```python
from build123d import *

# Parameters (mm, degrees)
SKETCH1_W           = 60
SKETCH1_H           = 54
BOSS_EXTRUDE1_DEPTH = 38
SKETCH2_W           = 44
SKETCH2_H           = 52
CUT_EXTRUDE1_DEPTH  = 19
SKETCH3_W           = 35
SKETCH3_H           = 52
CUT_EXTRUDE2_DEPTH  = 18
SKETCH4_W           = 6
SKETCH4_H           = 10
CUT_EXTRUDE3_DEPTH  = 38
SKETCH5_W           = 14
SKETCH5_H           = 52
CUT_EXTRUDE5_DEPTH  = 15
SKETCH6_W           = 13
SKETCH6_H           = 52
CUT_EXTRUDE6_DEPTH  = 4
SKETCH8_W           = 15
SKETCH8_H           = 13
CUT_EXTRUDE7_DEPTH  = 6
SKETCH10_W          = 13
SKETCH10_H          = 5
CUT_EXTRUDE8_DEPTH  = 6
SKETCH11_W          = 4
SKETCH11_H          = 5
CUT_EXTRUDE9_DEPTH  = 3
SKETCH12_W          = 5
SKETCH12_H          = 2
CUT_EXTRUDE10_DEPTH = 13
CUT_EXTRUDE11_DEPTH = 1
SKETCH14_W          = 13
SKETCH14_H          = 1
BOSS_EXTRUDE2_DEPTH = 4
SKETCH15_W          = 13
SKETCH15_H          = 1
BOSS_EXTRUDE3_DEPTH = 4


with BuildPart() as part:
    # Sketch1 → Boss-Extrude1 (new body)
    with BuildSketch(Plane(origin=(0, 0, 0), x_dir=(1, 0, 0), z_dir=(0, 1, 0))):
        with Locations((-83.874465942, -33.946435202)):
            Rectangle(SKETCH1_W, SKETCH1_H)
    extrude(amount=BOSS_EXTRUDE1_DEPTH)

    # Sketch2 → Cut-Extrude1 (cut)
    with BuildSketch(Plane(origin=(0, 38, 0), x_dir=(1, 0, 0), z_dir=(0, 1, 0))):
        with Locations((-76.874465942, -33.946435202)):
            Rectangle(SKETCH2_W, SKETCH2_H)
    extrude(amount=-CUT_EXTRUDE1_DEPTH, mode=Mode.SUBTRACT)

    # Sketch3 → Cut-Extrude2 (cut)
    with BuildSketch(Plane(origin=(0, 0, 0), x_dir=(-1, 0, 0), z_dir=(0, -1, 0))):
        with Locations((95.374465942, -33.946435202)):
            Rectangle(SKETCH3_W, SKETCH3_H)
    extrude(amount=-CUT_EXTRUDE2_DEPTH, mode=Mode.SUBTRACT)

    # Sketch4 → Cut-Extrude3 (cut)
    with BuildSketch(Plane(origin=(0, 18, 0), x_dir=(-1, 0, 0), z_dir=(0, -1, 0))):
        with Locations((108.874465942, -34.946435202)):
            Rectangle(SKETCH4_W, SKETCH4_H)
    extrude(amount=-CUT_EXTRUDE3_DEPTH, mode=Mode.SUBTRACT)

    # Sketch5 → Cut-Extrude5 (cut)
    with BuildSketch(Plane(origin=(0, 38, 0), x_dir=(1, 0, 0), z_dir=(0, 1, 0))):
        with Locations((-105.874465942, -33.946435202)):
            Rectangle(SKETCH5_W, SKETCH5_H)
    extrude(amount=-CUT_EXTRUDE5_DEPTH, mode=Mode.SUBTRACT)

    # Sketch6 → Cut-Extrude6 (cut)
    with BuildSketch(Plane(origin=(0, 23, 0), x_dir=(1, 0, 0), z_dir=(0, 1, 0))):
        with Locations((-106.374465942, -33.946435202)):
            Rectangle(SKETCH6_W, SKETCH6_H)
    extrude(amount=-CUT_EXTRUDE6_DEPTH, mode=Mode.SUBTRACT)

    # Sketch8 → Cut-Extrude7 (cut)
    with BuildSketch(Plane(origin=(0, 0, 0), x_dir=(-1, 0, 0), z_dir=(0, -1, 0))):
        with Locations((65.874465942, -17.946435202)):
            Rectangle(SKETCH8_W, SKETCH8_H)
    extrude(amount=-CUT_EXTRUDE7_DEPTH, mode=Mode.SUBTRACT)

    # Sketch10 → Cut-Extrude8 (cut)
    with BuildSketch(Plane(origin=(-73.374465942, 0, 0), x_dir=(0, 0, -1), z_dir=(1, 0, 0))):
        with Locations((-17.946435202, 3.5)):
            Rectangle(SKETCH10_W, SKETCH10_H)
    extrude(amount=-CUT_EXTRUDE8_DEPTH, mode=Mode.SUBTRACT)

    # Sketch11 → Cut-Extrude9 (cut)
    with BuildSketch(Plane.XZ):
        with Locations((-65.874465942, 48.446435202)):
            Rectangle(SKETCH11_W, SKETCH11_H)
    extrude(amount=-CUT_EXTRUDE9_DEPTH, mode=Mode.SUBTRACT)

    # Sketch12 → Cut-Extrude10 (cut)
    with BuildSketch(Plane(origin=(-67.874465942, 0, 0), x_dir=(0, 0, -1), z_dir=(1, 0, 0))):
        with Locations((-48.446435202, 2)):
            Rectangle(SKETCH12_W, SKETCH12_H)
    extrude(amount=-CUT_EXTRUDE10_DEPTH, mode=Mode.SUBTRACT)

    # Sketch13 → Cut-Extrude11 (cut)
    with BuildSketch(Plane.ZY.offset(113.874465942)):
        with BuildLine():
            Line((32.733045904, 15), (32.733045904, 22))
            ThreePointArc((32.733045904, 22), (35.233045904, 24.5), (37.733045904, 22))
            Line((37.733045904, 22), (37.733045904, 15))
            ThreePointArc((37.733045904, 15), (35.233045904, 12.5), (32.733045904, 15))
        make_face()
    extrude(amount=-CUT_EXTRUDE11_DEPTH, mode=Mode.SUBTRACT)

    # Sketch14 → Boss-Extrude2 (add)
    with BuildSketch(Plane(origin=(0, 19, 0), x_dir=(1, 0, 0), z_dir=(0, 1, 0))):
        with Locations((-106.374465942, -40.446435202)):
            Rectangle(SKETCH14_W, SKETCH14_H)
    extrude(amount=BOSS_EXTRUDE2_DEPTH)

    # Sketch15 → Boss-Extrude3 (add)
    with BuildSketch(Plane(origin=(0, 19, 0), x_dir=(1, 0, 0), z_dir=(0, 1, 0))):
        with Locations((-106.374465942, -29.446435202)):
            Rectangle(SKETCH15_W, SKETCH15_H)
    extrude(amount=BOSS_EXTRUDE3_DEPTH)


solid = part.part
```
Work out the finished part from the listing and answer in its coordinate system (mm). A direction names the side the tool comes from. Give positions to 0.01 mm unless a question says otherwise; leave off trailing zeros. Order: outer loops, then holes, each group sorted by start corner. A loop starts at its lowest first (then second) coordinate and runs counter-clockwise, first axis right, second up. Notation, with made-up numbers: M 61.25,50 L 95.25,50 A20 ccw 95.25,56 Z; hole C -39,-15.75 d7. An arc over 180 degrees is marked long. Return JSON: item names as keys, results as strings.
1) Section C-C, the plane y = 27 is taken. Write down the section's boundary in (x, z).
Resolved:
{"outline": "M -113.87,6.95 L -53.87,6.95 L -53.87,60.95 L -113.87,60.95 Z; hole M -112.87,7.95 L -54.87,7.95 L -54.87,59.95 L -112.87,59.95 Z"}
2) Section D-D, the plane x = -79 is taken. Write down the section's boundary in (y, z).
Resolved:
{"outline": "M 0,6.95 L 38,6.95 L 38,7.95 L 19,7.95 L 19,59.95 L 38,59.95 L 38,60.95 L 0,60.95 L 0,59.95 L 18,59.95 L 18,7.95 L 0,7.95 Z"}
3) Section A-A, the plane z = 32 is taken. Write down the section's boundary in (x, y).
Resolved:
{"outline": "M -113.87,0 L -112.87,0 L -112.87,18 L -111.87,18 L -111.87,19 L -112.87,19 L -112.87,38 L -113.87,38 Z; M -105.87,18 L -77.87,18 L -77.87,0 L -53.87,0 L -53.87,38 L -54.87,38 L -54.87,19 L -98.87,19 L -98.87,23 L -99.87,23 L -99.87,19 L -105.87,19 Z"}
4) A tool of negligible diameter and unlimited length cuts with its end or side. For faces 5 (the flat face through (-99.874, 21, 19)), 6 (the flat face through (-71, 2, 50.946)), 7 (the flat face through (-77.874, 9, 34)), from which of +Z, -Z, +X, -X, +Y, -Y can it reach the whole face along a straight path? Write none if from no direction.
Resolved:
{"face 5": "+Y", "face 6": "none", "face 7": "-Y"}
5) Section B-B, the plane y = 21 is taken. Write down the section's boundary in (x, z), plus the area to 3 significant figures.
Resolved:
{"outline": "M -113.87,6.95 L -53.87,6.95 L -53.87,60.95 L -113.87,60.95 L -113.87,37.73 L -112.87,37.73 L -112.87,39.95 L -99.87,39.95 L -99.87,29.95 L -112.87,29.95 L -112.87,32.73 L -113.87,32.73 Z; hole M -112.87,7.95 L -99.87,7.95 L -99.87,28.95 L -112.87,28.95 Z; hole M -112.87,40.95 L -99.87,40.95 L -99.87,59.95 L -112.87,59.95 Z; hole M -98.87,7.95 L -54.87,7.95 L -54.87,59.95 L -98.87,59.95 Z", "area": "297 mm^2"}
6) Straight lines are drawn through the part: line 1 along Z through (x, y) = (-110, 22.5); line 2 along Z through (x, y) = (-71, 2); line 3 along X through (y, z) = (22.5, 16). For each, find the intervals that lie inside material, in ascending order. Write a range as [from, to].
Resolved:
{"line 1": "[6.95, 7.95], [28.95, 29.95], [39.95, 40.95], [59.95, 60.95]", "line 2": "[6.95, 11.45], [24.45, 45.95], [50.95, 60.95]", "line 3": "[-113.87, -112.87], [-99.87, -98.87], [-54.87, -53.87]"}
7) Each of these flat-tipped pins is pushed along its axis until it touches: pin 1 (13 mm diameter, centred on x = -74.5, z = 27.5, fed in from +Y); pin 2 (1 mm diameter, centred on x = -100.5, z = 45, fed in from -Y). Where does it stop, or does it pass through?
Resolved:
{"pin 1": "y = 19", "pin 2": "y = 18"}
8) For a pull along X with two mould halves and no side action, classify faces 1 (the flat face through (-53.874, 19, 34)), 2 (the cylindrical face through (-113.4, 12.5, 35.3)), 3 (the flat face through (-68, 3, 11.446)), 4 (the flat face through (-76, 1, 18)) as +X half, -X half, draft (parallel to the pull), parting line (faces both ways), or undercut.
Resolved:
{"face 1": "+X half", "face 2": "draft", "face 3": "undercut", "face 4": "undercut"}
